from build123d import *

# Parameters (mm, degrees)
SKETCH1_W           = 14
SKETCH1_H           = 14
BOSS_EXTRUDE1_DEPTH = 2
FILLET1_R           = 0.5
SKETCH2_R           = 1.25
CUT_EXTRUDE1_DEPTH  = 2


with BuildPart() as part:
    # Sketch1 → Boss-Extrude1 (new body)
    with BuildSketch(Plane(origin=(0, 0, 0), x_dir=(1, 0, 0), z_dir=(0, 1, 0))):
        with Locations((-77.166666667, 63)):
            Rectangle(SKETCH1_W, SKETCH1_H)
    extrude(amount=BOSS_EXTRUDE1_DEPTH)

    # Fillet1
    fillet1_edges = [part.edges().sort_by_distance(p)[0] for p in [
        (-70.166666667, 2, -63),
        (-77.166666667, 2, -70),
        (-84.166666667, 2, -63),
        (-77.166666667, 0, -70),
        (-70.166666667, 0, -63),
        (-77.166666667, 0, -56),
        (-84.166666667, 0, -63),
        (-77.166666667, 2, -56),
        (-84.166666667, 1, -70),
        (-70.166666667, 1, -70),
        (-70.166666667, 1, -56),
        (-84.166666667, 1, -56),
    ]]
    fillet(fillet1_edges, radius=FILLET1_R)

    # Sketch2 → Cut-Extrude1 (cut)
    with BuildSketch(Plane(origin=(0, 2, 0), x_dir=(1, 0, 0), z_dir=(0, 1, 0))):
        with Locations(Location((-77.166666667, 63, 0), (0, 0, 270))):
            Circle(SKETCH2_R)
    extrude(amount=-CUT_EXTRUDE1_DEPTH, mode=Mode.SUBTRACT)


solid = part.part
Read the model definition and answer for the solid it produces. Units are mm, in the model's axes. Give positions to 0.01 mm unless a question says otherwise; leave off trailing zeros. Write each loop counter-clockwise with the first axis right and the second up, starting at its lowest first coordinate (ties: lowest second). Pieces come first, ordered by that corner, then holes. Notation, with made-up numbers: (70.5, 82.25) -> (124.5, 82.25) arc R12 ccw to (124.5, 99.25) -> close; hole circle Ø6 at (6, 75.25). An arc over 180 degrees is marked (long way). Answer as a JSON object with one key per item and string values. Group by question number.
1) The mould has two halves that part along X. Classify faces 1 (the flat face through (-77, 0, -65)), 2 (the flat face through (-84.167, 1, -63)), 3 (the cylindrical face through (-78.276, 1.014, -62.423)): +X half, -X half, draft (parallel to the pull), parting line (faces both ways), or undercut.
2) Find section B-B (y = 1.3). Write down the section's boundary in (x, z), and give its area (3 significant figures).
3) Find section A-A (z = -63). Write down the section's boundary in (x, y), and give its area (3 significant figures).
4) Consider L1, parallel to X at y = 1.15, z = -63; L2, parallel to Z at x = -78.25, y = 0.5; L3, parallel to Z at x = -72, y = 1.7. Determine where each line is inside the solid, lowest interval first. Write a range as from..to.
5) This flat-tipped pin is pushed along its axis until it touches: P1, Ø1.5, axis at x = -77.17, z = -63, coming from the +Y side. Where does it stop, or does it pass through?
Values follow:
{
 "1": {"face 1": "draft", "face 2": "-X half", "face 3": "undercut"},
 "2": {"outline": "(-84.17, -69.5) arc R0.5 ccw to (-83.67, -70) -> (-70.67, -70) arc R0.5 ccw to (-70.17, -69.5) -> (-70.17, -56.5) arc R0.5 ccw to (-70.67, -56) -> (-83.67, -56) arc R0.5 ccw to (-84.17, -56.5) -> close; hole circle Ø2.5 at (-77.17, -63)", "area": "191 mm2"},
 "3": {"outline": "(-84.17, 0.5) arc R0.5 ccw to (-83.67, 0) -> (-78.42, 0) -> (-78.42, 2) -> (-83.67, 2) arc R0.5 ccw to (-84.17, 1.5) -> close; (-75.92, 0) -> (-70.67, 0) arc R0.5 ccw to (-70.17, 0.5) -> (-70.17, 1.5) arc R0.5 ccw to (-70.67, 2) -> (-75.92, 2) -> close", "area": "22.8 mm2"},
 "4": {"L1": "x = -84.17..-78.42, -75.92..-70.17", "L2": "z = -70..-63.62, -62.38..-56", "L3": "z = -69.96..-56.04"},
 "5": {"P1": "passes through"}
}
